For this review, use the dimensioned drawing (mm, ordinates from the lowest corner) and the shaded views. Round coordinates to 2 decimals unless told otherwise and drop trailing zeros. Order: outer loops, then holes, each group sorted by start corner. A loop starts at its lowest first (then second) coordinate and runs counter-clockwise, first axis right, second up. Notation, with made-up numbers: M 79,10.5 L 136,10.5 A11 ccw 136,29.5 Z; hole C 19,31 d9. An arc over 180 degrees is marked long. Put each result on its own line as item: value.
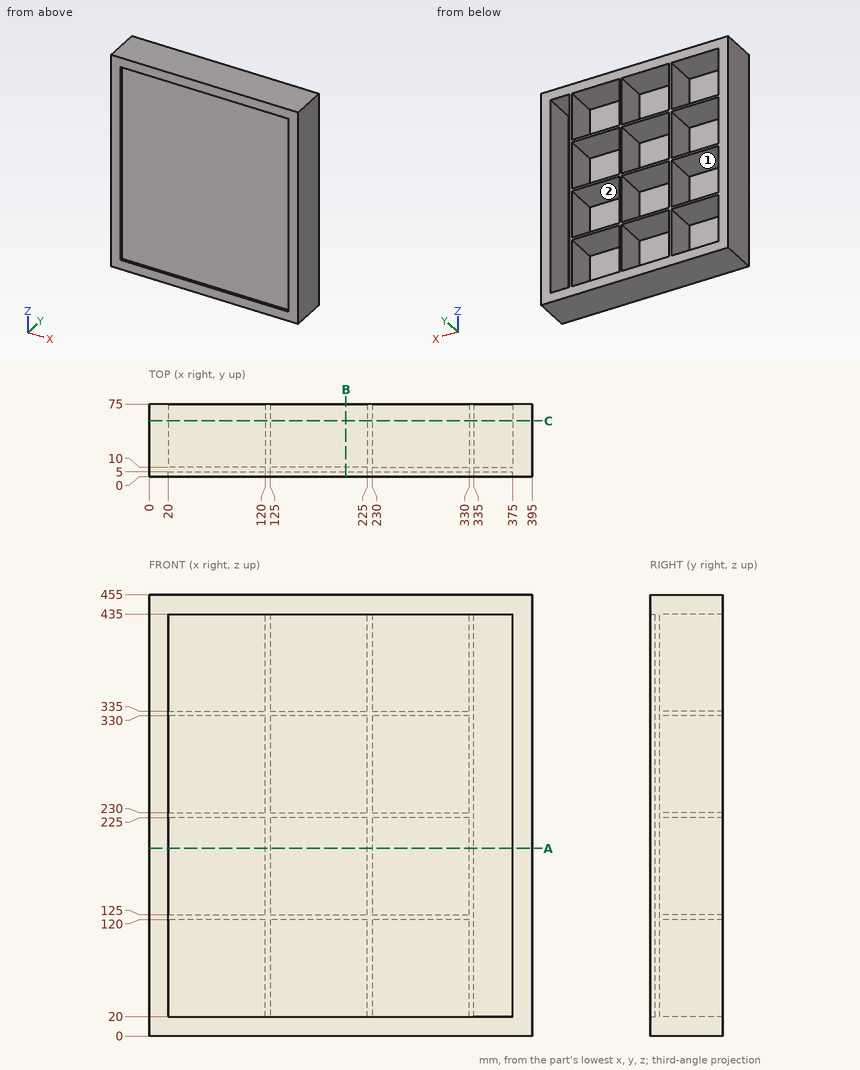
(1) Add section B-B on x = 203. Give the boundary of the cut face in (y, z).
A:
outline: M 0,0 L 75,0 L 75,20 L 10,20 L 10,120 L 75,120 L 75,125 L 10,125 L 10,225 L 75,225 L 75,230 L 10,230 L 10,330 L 75,330 L 75,335 L 10,335 L 10,435 L 75,435 L 75,455 L 0,455 L 0,435 L 5,435 L 5,20 L 0,20 Z
(2) Add section C-C on y = 57.5. State how many separate pieces and enclosed holes the cut face has, then the cut area to 3 significant figures.
A:
separate pieces: 1
enclosed holes: 13
area: 43,100 mm2
(3) Add section A-A on z = 193.5. Give the boundary of the cut face in (x, y), then the cut area to 3 significant figures.
A:
outline: M 0,0 L 20,0 L 20,5 L 375,5 L 375,0 L 395,0 L 395,75 L 375,75 L 375,10 L 335,10 L 335,75 L 330,75 L 330,10 L 230,10 L 230,75 L 225,75 L 225,10 L 125,10 L 125,75 L 120,75 L 120,10 L 20,10 L 20,75 L 0,75 Z
area: 5,750 mm2
(4) To check wall thickness, follow L1, parallel to X at y = 42, z = 403.5; L2, parallel to Z at x = 44, y = 58.5; L3, parallel to Z at x = 336.5, y = 69. State the ranges of each line that lie inside material, in increasing order.
A:
L1: x = 0 to 20, 120 to 125, 225 to 230, 330 to 335, 375 to 395
L2: z = 0 to 20, 120 to 125, 225 to 230, 330 to 335, 435 to 455
L3: z = 0 to 20, 435 to 455
(5) Insertion check: pin 1 Ø4 at (x, z) = (59, 252.5) entering from +Y; pin 2 Ø12 at (x, z) = (223.5, 55) entering from -Y. Each pin has a flat end and moves straight along its axis. Give the tip position at first contact, or say it passes through.
A:
pin 1: stops at y = 10
pin 2: stops at y = 5
(6) Draft analysis for pull direction Z (two halves, no side actions). For the marked faces 1 and 2, state which applies: released by +Z, released by -Z, zero draft, split by the parting line, or undercut.
A:
face 1: undercut
face 2: undercut
